Source: three-view drawing plus pictorial views. Frame: mm from the lowest corner of the part. Give positions to 0.01 mm unless a question says otherwise; leave off trailing zeros. Loops run counter-clockwise (first coordinate to the right, second up) from the corner with the lowest first, then second, coordinate; pieces in that order, holes last. Notation, with made-up numbers: (30.5, 63) - (64.5, 63) arc R13 cw to (64.5, 77) - close; hole circle Ø9 at (7, 42). An arc over 180 degrees is marked (long way). Write each question's results on one line, items separated by ' | '. Start each with the question number.
(1) Pull-direction query (X, two-part tool) for the marked faces 1, 2, 3 and 4; classes: pulls with the +X half, pulls with the -X half, needs draft (parallel to the pull), parting line crosses it, or undercut.
(2) Cut plane C-C on x = 43. Return the cut outline in (y, z).
(3) Material intervals for line 1 along Y through (x, z) = (43, 2.35); line 2 along X through (y, z) = (27, 3.4) (1 decimal); line 3 along X through (y, z) = (51.5, 3.5), sorted ascending. Write a range as [from, to].
(4) Cut plane B-B on z = 2.7. Return the cut outline in (x, y) (1 decimal), then the cut area to 3 significant figures.
(5) Cut plane D-D on y = 48.5. Return the cut outline in (x, z), then the cut area to 3 significant figures.
(6) Cut plane A-A on y = 35. Return the cut outline in (x, z).
(7) Contact query for flat-ended pins moving along their axis: pin 1 (1.5 mm diameter, centred on y = 32, z = 1.5, fed in from -X); pin 2 (1 mm diameter, centred on y = 59.5, z = 4, fed in from -X); pin 3 (2 mm diameter, centred on x = 11, z = 2, fed in from -Y). Output: stop coordinate, or through.
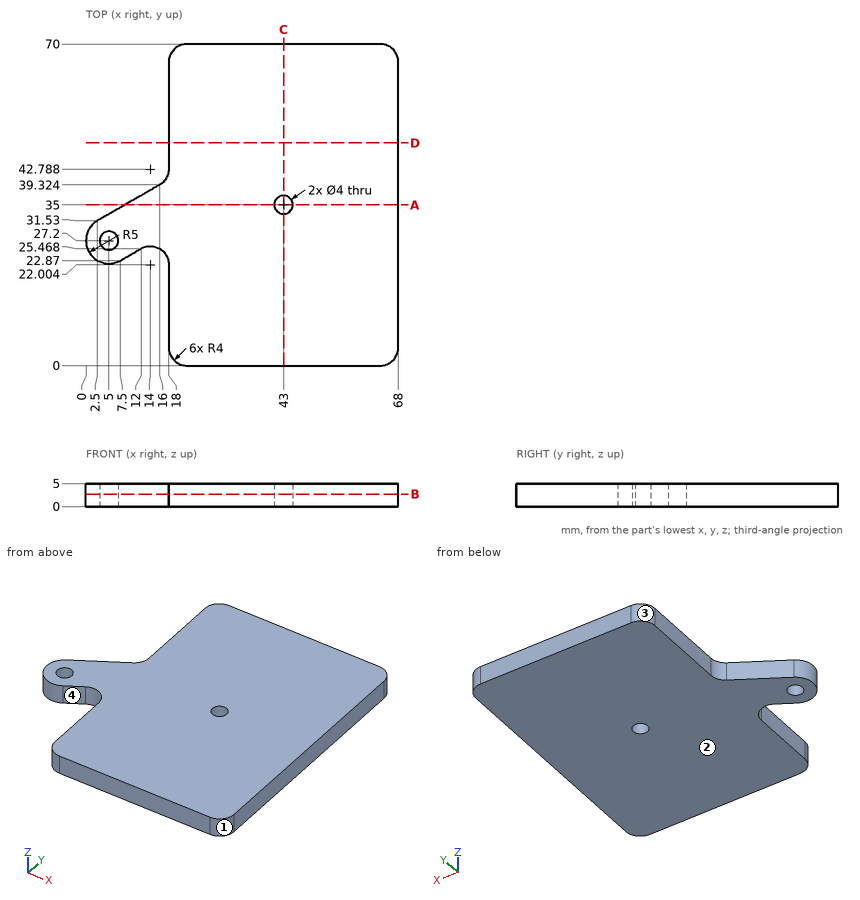
Ans:
1) face 1: pulls with the +X half | face 2: needs draft | face 3: pulls with the -X half | face 4: undercut
2) outline: (0, 0) - (33, 0) - (33, 5) - (0, 5) - close; (37, 0) - (70, 0) - (70, 5) - (37, 5) - close
3) line 1: [0, 33], [37, 70] | line 2: [0, 3], [7, 68] | line 3: [18, 68]
4) outline: (2.5, 31.5) arc R5 ccw to (7.5, 22.9) - (12, 25.5) arc R4 cw to (18, 22) - (18, 4) arc R4 ccw to (22, 0) - (64, 0) arc R4 ccw to (68, 4) - (68, 66) arc R4 ccw to (64, 70) - (22, 70) arc R4 ccw to (18, 66) - (18, 42.8) arc R4 cw to (16, 39.3) - close; hole circle Ø4 at (5, 27.2); hole circle Ø4 at (43, 35) | area: 3,660 mm^2
5) outline: (18, 0) - (68, 0) - (68, 5) - (18, 5) - close | area: 250 mm^2
6) outline: (8.51, 0) - (41, 0) - (41, 5) - (8.51, 5) - close; (45, 0) - (68, 0) - (68, 5) - (45, 5) - close
7) pin 1: x = 2.07 | pin 2: x = 18 | pin 3: y = 24.31
